```python
from build123d import *

# Parameters (mm, degrees)
BOSS_EXTRUDE1_DEPTH = 6
SKETCH2_R           = 3
CUT_EXTRUDE1_DEPTH  = 236.289183772
BOSS_EXTRUDE2_START = -6
BOSS_EXTRUDE2_DEPTH = 6


with BuildPart() as part:
    # Sketch1 → Boss-Extrude1 (new body)
    with BuildSketch(Plane.XY):
        with BuildLine():
            Line((-10, 0), (-10, 225))
            ThreePointArc((-10, 225), (0, 235), (10, 225))
            Line((10, 225), (10, 0))
            ThreePointArc((10, 0), (0, -10), (-10, 0))
        make_face()
    extrude(amount=BOSS_EXTRUDE1_DEPTH)

    # Sketch2 → Cut-Extrude1 (cut, through all)
    with BuildSketch(Plane.XY.offset(6)):
        with Locations((0, 225)):
            Circle(SKETCH2_R)
        Circle(SKETCH2_R)
    extrude(amount=-CUT_EXTRUDE1_DEPTH, mode=Mode.SUBTRACT)

    # Sketch3 → Boss-Extrude2 (add)
    with BuildSketch(Plane.XY.offset(6).offset(BOSS_EXTRUDE2_START)):
        with BuildLine():
            Line((-10, 225), (-10, 265))
            ThreePointArc((-10, 265), (0, 275), (10, 265))
            Line((10, 265), (10, 225))
            ThreePointArc((10, 225), (0, 235), (-10, 225))
        make_face()
    extrude(amount=BOSS_EXTRUDE2_DEPTH)


solid = part.part
```
Part model, mm, in its own coordinate system. Coordinates: 2 decimals unless noted, no trailing zeros. Order: outer loops, then holes, each group sorted by start corner. A loop starts at its lowest first (then second) coordinate and runs counter-clockwise, first axis right, second up. Notation, with made-up numbers: (56.5, 54.5) - (105.5, 54.5) arc R16 ccw to (105.5, 78.5) - close; hole circle Ø3 at (62.5, -22.5). An arc over 180 degrees is marked (long way). Return JSON: item names as keys, results as strings. Group by question number.
Item 1: Pin check, flat tip, straight feed: pin 1 (1.5 mm diameter, centred on x = -5.5, z = 1.5, fed in from +Y). Stop position of the tip, or through.
Item 2: Cut at A-A (y = 225). List the corners of the cut face in (x, z), plus the area to 3 significant figures.
Item 3: Cut at B-B (z = 2.5). List the corners of the cut face in (x, y).
Item 4: Pull direction Y, two halves, no side cores. Call faces 1 (the face through (-3, 0, 3)), 2 (the face through (0, -10, 3)), 3 (the face through (0, 275, 3)), 4 (the face through (-10, 131, 3)): pulls with the +Y half, pulls with the -Y half, needs draft (parallel to the pull), parting line crosses it, or undercut.
Item 5: Drill centre lines: probe 1 along Y at (x, z) = (0, 3.75); probe 2 along Y at (x, z) = (1.25, 2.35); probe 3 along X at (y, z) = (225, 1.9). Where is each one in solid material? Low to high. Write a range as from..to.
Item 6: Cut at C-C (x = 7.25). List the corners of the cut face in (y, z), plus the area to 3 significant figures.
Check values:
{
 "1": {"pin 1": "stops at y = 273.8"},
 "2": {"outline": "(-10, 0) - (-3, 0) - (-3, 6) - (-10, 6) - close; (3, 0) - (10, 0) - (10, 6) - (3, 6) - close", "area": "84.0 mm2"},
 "3": {"outline": "(-10, 0) arc R10 ccw to (10, 0) - (10, 265) arc R10 ccw to (-10, 265) - close; hole circle Ø6 at (0, 0); hole circle Ø6 at (0, 225)"},
 "4": {"face 1": "undercut", "face 2": "pulls with the -Y half", "face 3": "pulls with the +Y half", "face 4": "needs draft"},
 "5": {"probe 1": "y = -10..-3, 3..222, 228..275", "probe 2": "y = -9.92..-2.73, 2.73..222.27, 227.73..274.92", "probe 3": "x = -10..-3, 3..10"},
 "6": {"outline": "(-6.89, 0) - (271.89, 0) - (271.89, 6) - (-6.89, 6) - close", "area": "1,670 mm2"}
}
